Verification items for this drawing (mm, ordinates from the low corner). A direction names the side the tool comes from. Round coordinates to 2 decimals unless told otherwise and drop trailing zeros. Order: outer loops, then holes, each group sorted by start corner. A loop starts at its lowest first (then second) coordinate and runs counter-clockwise, first axis right, second up. Notation, with made-up numbers: M 7.25,-28.5 L 62.25,-28.5 A10 cw 62.25,-17.5 Z; hole C 7,32.25 d3. An arc over 180 degrees is marked long. Use CSV: the item, a comma, the result in double quotes. Start each with the question number.
Q1. Sectioned sample at A-A (x = 104). Enter the section's corners in (y, z).
Q2. Scan lines: line 1 (Z direction, x = 104, y = 46.65); line 2 (Y direction, x = 27, z = 8.5); line 3 (Z direction, x = 7, y = 6.5). Record each from-to range of solid material in increasing order.
Q3. Sectioned sample at D-D (y = 17). Enter the section's corners in (x, z), and give its area (4 significant figures).
Q4. Gauge pin test, flat ends, axial feed: pin 1 Ø13.5 at (x, y) = (55.5, 17.5) entering from -Z; pin 2 Ø3.5 at (x, y) = (46.5, 47) entering from +Z; pin 3 Ø1 at (x, z) = (28, 21) entering from -Y. Record the tip position at first contact, or that the pin passes through.
Q5. Sectioned sample at C-C (x = 34). Enter the section's corners in (y, z).
Q6. Set-up check for the marked faces 1, 2 and 3: record each of +Z, -Z, +X, -X, +Y, -Y from which the full face is reachable in a straight line by a thin tool's end or side.
Q7. Sectioned sample at B-B (z = 4). Enter the section's corners in (x, y), and give its area (4 significant figures).
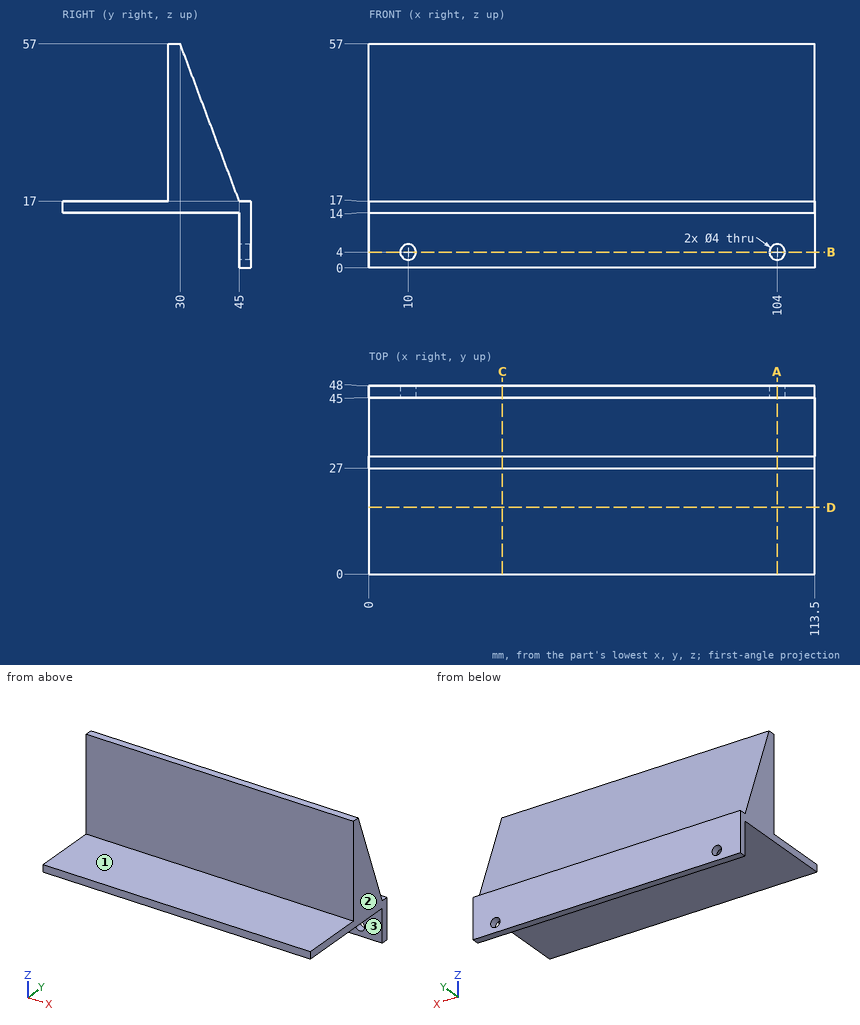
Verdict:
1,outline,"M 0,14 L 45,14 L 45,6 L 48,6 L 48,17 L 45,17 L 30,57 L 27,57 L 27,17 L 0,17 Z; M 45,0 L 48,0 L 48,2 L 45,2 Z"
2,line 1,"z = 0 to 2, 6 to 17"
2,line 2,"y = 45 to 48"
2,line 3,"z = 14 to 17"
3,outline,"M 0,14 L 113.5,14 L 113.5,17 L 0,17 Z"
3,area,"340.5 mm²"
4,pin 1,"stops at z = 14"
4,pin 2,"stops at z = 17"
4,pin 3,"stops at y = 27"
5,outline,"M 0,14 L 45,14 L 45,0 L 48,0 L 48,17 L 45,17 L 30,57 L 27,57 L 27,17 L 0,17 Z"
6,face 1,"+Z, +X, -X, -Y"
6,face 2,"+Z, -Z, +X, +Y, -Y"
6,face 3,"-Z, +X, -X, -Y"
7,outline,"M 0,45 L 8,45 L 8,48 L 0,48 Z; M 12,45 L 102,45 L 102,48 L 12,48 Z; M 106,45 L 113.5,45 L 113.5,48 L 106,48 Z"
7,area,"316.5 mm²"
